from build123d import *

# Parameters (mm, degrees)
F3_DEPTH      = 23
F3_DEPTH_BACK = 23
F2_W          = 71.3
F2_H          = 2.5
F2_W_2        = 160.6
F2_H_2        = 20
F2_W_3        = 155.6
F2_H_3        = 15
F2_W_4        = 150.6
F4_DEPTH      = 5
F7_DEPTH      = 95
F7_DEPTH_BACK = 95
F8_DEPTH      = 12
F8_DEPTH_BACK = 12
F9_DEPTH      = 4.75


# Not quite as in the source:
# - a feature names something its author has since deleted; it is built from what else it names


with BuildPart() as f3:
    # F0 (on Front) → F3 (new body, two sides)
    with BuildSketch(Plane.XZ) as f3_sk:
        with BuildLine():
            Line((0, 1.5), (0, 0))
            Line((0, 0), (1.5, 0))
            ThreePointArc((1.5, 0), (1.0606601718, 1.0606601718), (0, 1.5))
        make_face()
        with BuildLine():
            ThreePointArc((0, 1.5), (-1.0606601718, 1.0606601718), (-1.5, 0))
            Line((-1.5, 0), (0, 0))
            Line((0, 0), (0, 1.5))
        make_face()
        with BuildLine():
            Line((-91.6240630262, 0), (-79.4154876804, 0))
            Line((-79.4154876804, 0), (-1.5, 0))
            ThreePointArc((-1.5, 0), (-1.0606601718, 1.0606601718), (0, 1.5))
            Line((0, 1.5), (0, 4.75))
            ThreePointArc((0, 4.75), (-39.7521168613, 3.8147080292), (-79.4154876804, 1))
            Line((-79.4154876804, 1), (-91.6240630262, 4.75))
            Line((-91.6240630262, 4.75), (-91.6240630262, 0))
        make_face()
        with BuildLine():
            Line((0, 4.75), (0, 1.5))
            ThreePointArc((0, 1.5), (1.0606601718, 1.0606601718), (1.5, 0))
            Line((1.5, 0), (79.1845123196, 0))
            Line((79.1845123196, 0), (92.3759369738, 0))
            Line((92.3759369738, 0), (92.3759369738, 4.75))
            Line((92.3759369738, 4.75), (79.1845123196, 1))
            ThreePointArc((79.1845123196, 1), (39.6365002683, 3.8092528426), (0, 4.75))
        make_face()
    extrude(amount=F3_DEPTH)
    extrude(f3_sk.sketch, amount=-F3_DEPTH_BACK)

    # F2 (on Top) → F4 (cut)
    with BuildSketch(Plane.XY):
        with Locations((-39.65, -14.75)):
            Rectangle(F2_W, F2_H)
        with Locations((39.65, -14.75)):
            Rectangle(F2_W, F2_H)
        Rectangle(F2_W_2, F2_H_2)
        Rectangle(F2_W_3, F2_H_3, mode=Mode.SUBTRACT)
        with Locations((0, 15.5593407378)):
            Rectangle(F2_W_4, F2_H)
    extrude(amount=F4_DEPTH, mode=Mode.SUBTRACT)

    # F6 (on Right) → F7 (join, two sides)
    with BuildSketch(Plane.YZ) as f7_sk:
        with BuildLine():
            Line((-2, 0), (2, 0))
            ThreePointArc((2, 0), (0, 2), (-2, 0))
        make_face()
    extrude(amount=F7_DEPTH)
    extrude(f7_sk.sketch, amount=-F7_DEPTH_BACK)

    # F0 (on Front) → F8 (join, two sides)
    with BuildSketch(Plane.XZ) as f8_sk:
        with BuildLine():
            Line((0, 1.5), (0, 0))
            Line((0, 0), (1.5, 0))
            ThreePointArc((1.5, 0), (1.0606601718, 1.0606601718), (0, 1.5))
        make_face()
        with BuildLine():
            ThreePointArc((0, 1.5), (-1.0606601718, 1.0606601718), (-1.5, 0))
            Line((-1.5, 0), (0, 0))
            Line((0, 0), (0, 1.5))
        make_face()
    extrude(amount=F8_DEPTH)
    extrude(f8_sk.sketch, amount=-F8_DEPTH_BACK)

    # F2 (on Top) → F9 (join)
    with BuildSketch(Plane.XY):
        Rectangle(F2_W_3, F2_H_3)
    extrude(amount=F9_DEPTH)


solid = f3.part
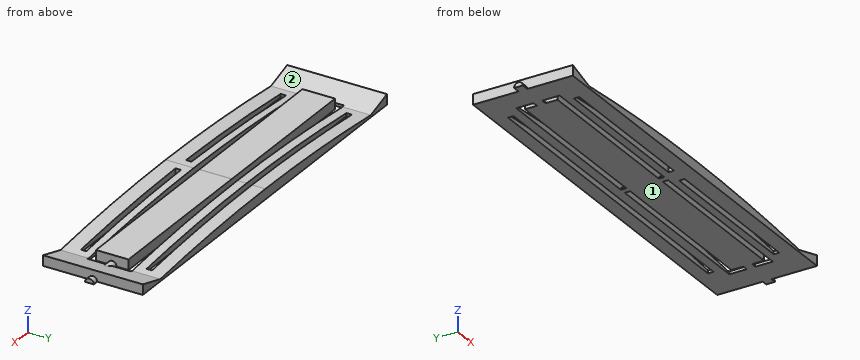
Build history of the part. All positions in model axes, mm. Face numbers are marked on the shaded views. Give positions to 0.01 mm unless a question says otherwise; leave off trailing zeros. Write each loop counter-clockwise with the first axis right and the second up, starting at its lowest first coordinate (ties: lowest second). Pieces come first, ordered by that corner, then holes. Notation, with made-up numbers: (80, -38.5) - (125, -38.5) arc R33 ccw to (125, -10.5) - close; hole circle Ø6 at (41, 59.25). An arc over 180 degrees is marked (long way). Use one line per item in the form item = value. Start each with the question number.
1. Band-saw the part on B-B on x = 56.5. Write the cut outline in (y, z).
2. Band-saw the part on C-C on x = 29.5. Write the cut outline in (y, z), plus the area to 3 significant figures.
3. Band-saw the part on A-A on y = 19.5. Write the cut outline in (x, z), plus the area to 3 significant figures.
4. Two-plate mould, pull along X, no slides. Class the marked faces 1 and 2: released by +X, released by -X, zero draft, split by the parting line, or undercut.
5. Drop a flat-ended pin along its axis: pin 1 Ø1.4 at (y, z) = (-4.5, 0.5) entering from +X. Give the stop position or say it passes through.
6. Probe line 1 (Y direction, x = 73, z = 0.55); line 2 (X direction, y = 7, z = 0.5); line 3 (X direction, y = 17.5, z = 0.45). List the from-to ranges inside material, lowest first. Write a range as [from, to].
Conclusion:
q1.outline = (-23, 0) - (-16, 0) - (-16, 2.84) - (-23, 2.84) - close; (-13.5, 0) - (-10, 0) - (-10, 2.84) - (-13.5, 2.84) - close; (-7.5, 0) - (7.5, 0) - (7.5, 4.75) - (-7.5, 4.75) - close; (10, 0) - (14.31, 0) - (14.31, 2.84) - (10, 2.84) - close; (16.81, 0) - (23, 0) - (23, 2.84) - (16.81, 2.84) - close
q2.outline = (-23, 0) - (-16, 0) - (-16, 4.23) - (-23, 4.23) - close; (-13.5, 0) - (-10, 0) - (-10, 4.23) - (-13.5, 4.23) - close; (-7.5, 0) - (7.5, 0) - (7.5, 4.75) - (-7.5, 4.75) - close; (10, 0) - (14.31, 0) - (14.31, 4.23) - (10, 4.23) - close; (16.81, 0) - (23, 0) - (23, 4.23) - (16.81, 4.23) - close
q2.area = 160 mm²
q3.outline = (-91.62, 0) - (92.38, 0) - (92.38, 4.75) - (79.18, 1) arc R840.34 ccw to (-79.42, 1) - (-91.62, 4.75) - close
q3.area = 628 mm²
q4.face_1 = zero draft
q4.face_2 = undercut
q5.pin_1 = 92.38
q6.line_1 = [-23, -16], [-13.5, -10], [-7.5, 7.5], [10, 14.31], [16.81, 23]
q6.line_2 = [-91.62, -80.3], [-77.8, 77.8], [80.3, 92.38]
q6.line_3 = [-91.62, 92.38]
